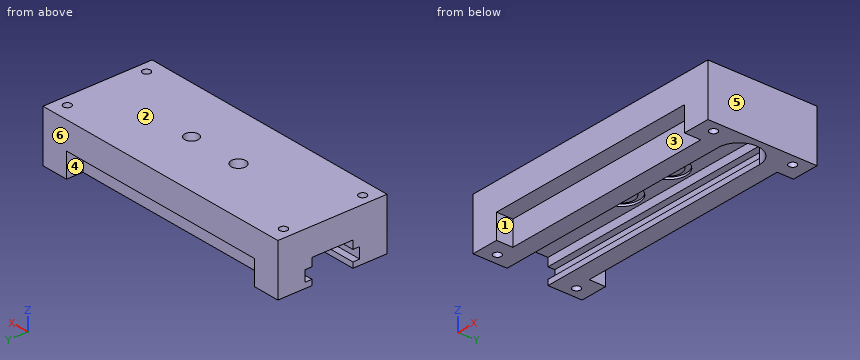
from build123d import *

# Parameters (mm, degrees)
SKETCH1_W           = 100
SKETCH1_H           = 40
BOSS_EXTRUDE1_DEPTH = 38
CUT_EXTRUDE4_REACH  = 81.36
SKETCH4_R           = 1.45
SKETCH6_W           = 100
SKETCH6_H           = 19
CUT_EXTRUDE5_DEPTH  = 87.215210375
CUT_EXTRUDE12_DEPTH = 9
CUT_EXTRUDE13_REACH = 72.385
SKETCH18_R          = 2.506862912
SKETCH18_R_2        = 2.693115416
SKETCH19_R          = 6.477
SKETCH19_R_2        = 4.572
CUT_EXTRUDE14_DEPTH = 0.79375
SKETCH21_W          = 10
SKETCH21_H          = 15
CUT_EXTRUDE15_DEPTH = 9
SKETCH22_W          = 4
SKETCH22_H          = 2.5
CUT_EXTRUDE16_DEPTH = 90
SKETCH23_W          = 80
SKETCH23_H          = 6
CUT_EXTRUDE17_DEPTH = 9


with BuildPart() as part:
    # Sketch1 → Boss-Extrude1 (new body)
    with BuildSketch(Plane.XY):
        with Locations((16.25, 1.5625)):
            Rectangle(SKETCH1_W, SKETCH1_H)
    extrude(amount=BOSS_EXTRUDE1_DEPTH)

    # Sketch4 → Cut-Extrude4 (cut, up to next)
    with BuildSketch(Plane(origin=(0, 0, 0), x_dir=(-1, 0, 0), z_dir=(0, 0, -1)), mode=Mode.PRIVATE) as cut_extrude4_sk1:
        with Locations((-62.25, 16.0625)):
            Circle(SKETCH4_R)
    cut_extrude4_tool1 = extrude(cut_extrude4_sk1.sketch, amount=-CUT_EXTRUDE4_REACH, mode=Mode.PRIVATE) & part.part
    # Sketch4 → Cut-Extrude4 (cut, up to next)
    with BuildSketch(Plane(origin=(0, 0, 0), x_dir=(-1, 0, 0), z_dir=(0, 0, -1)), mode=Mode.PRIVATE) as cut_extrude4_sk2:
        with Locations((-62.25, -12.9375)):
            Circle(SKETCH4_R)
    cut_extrude4_tool2 = extrude(cut_extrude4_sk2.sketch, amount=-CUT_EXTRUDE4_REACH, mode=Mode.PRIVATE) & part.part
    # Sketch4 → Cut-Extrude4 (cut, up to next)
    with BuildSketch(Plane(origin=(0, 0, 0), x_dir=(-1, 0, 0), z_dir=(0, 0, -1)), mode=Mode.PRIVATE) as cut_extrude4_sk3:
        with Locations((29.75, 16.0625)):
            Circle(SKETCH4_R)
    cut_extrude4_tool3 = extrude(cut_extrude4_sk3.sketch, amount=-CUT_EXTRUDE4_REACH, mode=Mode.PRIVATE) & part.part
    # Sketch4 → Cut-Extrude4 (cut, up to next)
    with BuildSketch(Plane(origin=(0, 0, 0), x_dir=(-1, 0, 0), z_dir=(0, 0, -1)), mode=Mode.PRIVATE) as cut_extrude4_sk4:
        with Locations((29.75, -12.9375)):
            Circle(SKETCH4_R)
    cut_extrude4_tool4 = extrude(cut_extrude4_sk4.sketch, amount=-CUT_EXTRUDE4_REACH, mode=Mode.PRIVATE) & part.part
    add(cut_extrude4_tool1.solids().sort_by_distance((62.25, 16.0625, 0))[0], mode=Mode.SUBTRACT)
    add(cut_extrude4_tool2.solids().sort_by_distance((62.25, -12.9375, 0))[0], mode=Mode.SUBTRACT)
    add(cut_extrude4_tool3.solids().sort_by_distance((-29.75, 16.0625, 0))[0], mode=Mode.SUBTRACT)
    add(cut_extrude4_tool4.solids().sort_by_distance((-29.75, -12.9375, 0))[0], mode=Mode.SUBTRACT)

    # Sketch6 → Cut-Extrude5 (cut, through all)
    with BuildSketch(Plane(origin=(0, 21.5625, 0), x_dir=(1, 0, 0), z_dir=(0, 1, 0))):
        with Locations((16.25, -28.5)):
            Rectangle(SKETCH6_W, SKETCH6_H)
    extrude(amount=-CUT_EXTRUDE5_DEPTH, mode=Mode.SUBTRACT)

    # Sketch17 → Cut-Extrude12 (cut)
    with BuildSketch(Plane(origin=(0, 0, 0), x_dir=(-1, 0, 0), z_dir=(0, 0, -1))):
        with BuildLine():
            Line((-56.25, 9.0625), (23.75, 9.0625))
            ThreePointArc((23.75, 9.0625), (31.25, 1.5625), (23.75, -5.9375))
            Line((23.75, -5.9375), (-56.25, -5.9375))
            ThreePointArc((-56.25, -5.9375), (-63.75, 1.5625), (-56.25, 9.0625))
        make_face()
    extrude(amount=-CUT_EXTRUDE12_DEPTH, mode=Mode.SUBTRACT)

    # Sketch18 → Cut-Extrude13 (cut, up to next)
    with BuildSketch(Plane(origin=(0, 0, 9), x_dir=(-1, 0, 0), z_dir=(0, 0, -1)), mode=Mode.PRIVATE) as cut_extrude13_sk1:
        with Locations((-26.25, 1.5625)):
            Circle(SKETCH18_R)
    cut_extrude13_tool1 = extrude(cut_extrude13_sk1.sketch, amount=-CUT_EXTRUDE13_REACH, mode=Mode.PRIVATE) & part.part
    # Sketch18 → Cut-Extrude13 (cut, up to next)
    with BuildSketch(Plane(origin=(0, 0, 9), x_dir=(-1, 0, 0), z_dir=(0, 0, -1)), mode=Mode.PRIVATE) as cut_extrude13_sk2:
        with Locations((-6.25, 1.5625)):
            Circle(SKETCH18_R_2)
    cut_extrude13_tool2 = extrude(cut_extrude13_sk2.sketch, amount=-CUT_EXTRUDE13_REACH, mode=Mode.PRIVATE) & part.part
    add(cut_extrude13_tool1.solids().sort_by_distance((26.25, 1.5625, 9))[0], mode=Mode.SUBTRACT)
    add(cut_extrude13_tool2.solids().sort_by_distance((6.25, 1.5625, 9))[0], mode=Mode.SUBTRACT)

    # Sketch19 → Cut-Extrude14 (cut)
    # profile 1 of 2: a face of its own
    with BuildSketch(Plane(origin=(0, 0, 9), x_dir=(-1, 0, 0), z_dir=(0, 0, -1))):
        with Locations((-26.25, 1.5625)):
            Circle(SKETCH19_R)
        with Locations((-26.25, 1.5625)):
            Circle(SKETCH19_R_2, mode=Mode.SUBTRACT)
    # profile 2 of 2: a face of its own
    with BuildSketch(Plane(origin=(0, 0, 9), x_dir=(-1, 0, 0), z_dir=(0, 0, -1))):
        with Locations((-6.25, 1.5625)):
            Circle(SKETCH19_R)
        with Locations((-6.25, 1.5625)):
            Circle(SKETCH19_R_2, mode=Mode.SUBTRACT)
    extrude(amount=-CUT_EXTRUDE14_DEPTH, mode=Mode.SUBTRACT)

    # Sketch21 → Cut-Extrude15 (cut)
    with BuildSketch(Plane(origin=(0, 0, 0), x_dir=(-1, 0, 0), z_dir=(0, 0, -1))):
        with Locations((28.75, 1.5625)):
            Rectangle(SKETCH21_W, SKETCH21_H)
    extrude(amount=-CUT_EXTRUDE15_DEPTH, mode=Mode.SUBTRACT)

    # Sketch22 → Cut-Extrude16 (cut)
    with BuildSketch(Plane.ZY.offset(33.75)):
        with Locations((4, 10.3125)):
            Rectangle(SKETCH22_W, SKETCH22_H)
        with Locations((4, -7.1875)):
            Rectangle(SKETCH22_W, SKETCH22_H)
    extrude(amount=-CUT_EXTRUDE16_DEPTH, mode=Mode.SUBTRACT)

    # Sketch23 → Cut-Extrude17 (cut)
    with BuildSketch(Plane(origin=(0, 0, 0), x_dir=(-1, 0, 0), z_dir=(0, 0, -1))):
        with Locations((-16.25, 18.5625)):
            Rectangle(SKETCH23_W, SKETCH23_H)
        with Locations((-16.25, -15.4375)):
            Rectangle(SKETCH23_W, SKETCH23_H)
    extrude(amount=-CUT_EXTRUDE17_DEPTH, mode=Mode.SUBTRACT)


solid = part.part
Work out the finished part from the listing and answer in its coordinate system (mm). Face numbers are marked on the shaded views. A direction names the side the tool comes from. Coordinates: 2 decimals unless noted, no trailing zeros. Write each loop counter-clockwise with the first axis right and the second up, starting at its lowest first coordinate (ties: lowest second). Pieces come first, ordered by that corner, then holes.
1. For the marked faces 1 and 2, determine the directions among +Z, -Z, +X, -X, +Y, -Y from which every point of the face is accessible in a straight line to the end or side of a thin tool.
Results list:
face 1: -Z, -Y
face 2: +Z, +X, -X, +Y, -Y
2. The part is cut by section A-A, the plane x = -29.75. Write down the section's boundary in (y, z), and give its area (3 significant figures).
Results list:
outline: (-18.44, 0) - (-14.39, 0) - (-14.39, 19) - (-18.44, 19) - close; (-11.49, 0) - (-5.94, 0) - (-5.94, 2) - (-8.44, 2) - (-8.44, 6) - (-5.94, 6) - (-5.94, 9) - (9.06, 9) - (9.06, 6) - (11.56, 6) - (11.56, 2) - (9.06, 2) - (9.06, 0) - (14.61, 0) - (14.61, 19) - (-11.49, 19) - close; (17.51, 0) - (21.56, 0) - (21.56, 19) - (17.51, 19) - close
area: 495 mm2
3. The part is cut by section D-D, the plane x = 46. Write down the section's boundary in (y, z), and give its area (3 significant figures).
Results list:
outline: (-18.44, 9) - (-12.44, 9) - (-12.44, 0) - (-5.94, 0) - (-5.94, 2) - (-8.44, 2) - (-8.44, 6) - (-5.94, 6) - (-5.94, 9) - (9.06, 9) - (9.06, 6) - (11.56, 6) - (11.56, 2) - (9.06, 2) - (9.06, 0) - (15.56, 0) - (15.56, 9) - (21.56, 9) - (21.56, 19) - (-18.44, 19) - close
area: 497 mm2
4. Consider line 1 along Y through (x, z) = (6.25, 9.6); line 2 along Y through (x, z) = (62.25, 11); line 3 along Z through (x, y) = (23, 11.5). Determine where each line is inside the solid, lowest interval first.
Results list:
line 1: y = -18.44 to -4.91, -3.01 to -1.13, 4.26 to 6.13, 8.04 to 21.56
line 2: y = -18.44 to -14.39, -11.49 to 14.61, 17.51 to 21.56
line 3: z = 0 to 2, 6 to 19
5. Flat-ended cylindrical pins translate along their axes: pin 1 (2.5 mm diameter, centred on x = -4.5, z = 7, fed in from +Y); pin 2 (0.8 mm diameter, centred on y = 10, z = 4.5, fed in from -X); pin 3 (2 mm diameter, centred on x = 29, z = 1, fed in from -Y). Find the tip coordinate at first contact, or state that the pin passes through.
Results list:
pin 1: stops at y = 15.56
pin 2: stops at x = 56.25
pin 3: stops at y = -12.44
6. The part is cut by section C-C, the plane z = 15. Write down the section's boundary in (x, y), and give its area (3 significant figures).
Results list:
outline: (-33.75, -18.44) - (66.25, -18.44) - (66.25, 21.56) - (-33.75, 21.56) - close; hole circle Ø2.9 at (-29.75, -12.94); hole circle Ø2.9 at (-29.75, 16.06); hole circle Ø5.39 at (6.25, 1.56); hole circle Ø5.01 at (26.25, 1.56); hole circle Ø2.9 at (62.25, -12.94); hole circle Ø2.9 at (62.25, 16.06)
area: 3,930 mm2
7. For a pull along X with two mould halves and no side action, classify the marked faces 3, 4, 5 and 6 as +X half, -X half, draft (parallel to the pull), parting line (faces both ways), or undercut.
Results list:
face 3: undercut
face 4: undercut
face 5: +X half
face 6: draft
